Read the model definition and answer for the solid it produces. Units are mm, in the model's axes. Face numbers are marked on the shaded views. A direction names the side the tool comes from. Coordinates: 2 decimals unless noted, no trailing zeros. Order: outer loops, then holes, each group sorted by start corner. A loop starts at its lowest first (then second) coordinate and runs counter-clockwise, first axis right, second up. Notation, with made-up numbers: (-37, -7) -> (13, -7) arc R27 cw to (13, 28) -> close; hole circle Ø4 at (72, 86.5). An arc over 180 degrees is marked (long way). Answer as a JSON object with one key per item and string values. Group by question number.
1) Consider L1, parallel to X at y = -4.5, z = 1.95; L2, parallel to Y at x = 0, z = 1.3; L3, parallel to Y at x = 0, z = 4.2. Determine where each line is inside the solid, lowest interval first.
2) A tool of negligible diameter and unlimited length cuts with its end or side. For the marked faces 1 and 2, from which of +Z, -Z, +X, -X, +Y, -Y can it reach the whole face along a straight path? Write none if from no direction.
3) Section C-C on z = 2 is taken. Determine the outline of the cut face in (x, y), and give its area (3 significant figures).
4) Section D-D on y = -4.75 is taken. Determine the outline of the cut face in (x, z).
5) Determine the mould class of the marked faces 3, 4 and 5 for opening direction Z: released by +Z, released by -Z, zero draft, split by the parting line, or undercut.
6) Section B-B on y = 0 is taken. Determine the outline of the cut face in (x, z), and give its area (3 significant figures).
7) Section A-A on x = 0 is taken. Determine the outline of the cut face in (y, z), and give its area (3 significant figures).
8) Given pin 1 (2.5 mm diameter, centred on x = 2, y = 2, fed in from -Z), flat-ended and moving along its own axis, determine where the tip first touches the part or whether it passes through.
from build123d import *

# Parameters (mm, degrees)
ESBO_O6_R                  = 5.25
ESBO_O6_R_2                = 4.1
RESSALTO_EXTRUS_O3_DEPTH   = 4
ESBO_O7_R                  = 5.25
RESSALTO_EXTRUS_O4_DEPTH   = 0.5
ESBO_O9_R                  = 0.65
RESSALTO_EXTRUS_O5_DEPTH   = 1.2
ESBO_O12_R                 = 3
CORTE_EXTRUS_O5_DEPTH      = 10
RESSALTO_EXTRUS_O6_START   = 4
ESBO_O13_R                 = 4.1
ESBO_O13_R_2               = 3.85
RESSALTO_EXTRUS_O6_DEPTH   = 4
ESBO_O16_W                 = 2.665336127
ESBO_O16_H                 = 7.90902753
ESBO_O16_W_2               = 2.097265449
ESBO_O16_H_2               = 7.395164159
CORTE_EXTRUS_O7_DEPTH      = 10
ESBO_O15_W                 = 9
ESBO_O15_H                 = 11
ESBO_O15_R                 = 3.85
RESSALTO_EXTRUS_O7_DEPTH   = 4.5
CORTE_EXTRUS_O6_REACH      = 18.756
CORTE_EXTRUS_O6_END_RADIUS = 3.85
ESBO_O14_R                 = 0.5


with BuildPart() as part:
    # Esboço6 → Ressalto-extrusão3 (new body)
    with BuildSketch(Plane.XY):
        Circle(ESBO_O6_R)
        Circle(ESBO_O6_R_2, mode=Mode.SUBTRACT)
    extrude(amount=RESSALTO_EXTRUS_O3_DEPTH)

    # Esboço7 → Ressalto-extrusão4 (add)
    with BuildSketch(Plane.XY.offset(4)):
        Circle(ESBO_O7_R)
    extrude(amount=RESSALTO_EXTRUS_O4_DEPTH)

    # Esboço9 → Ressalto-extrusão5 (add)
    with BuildSketch(Plane(origin=(0, 0, 0), x_dir=(-1, 0, 0), z_dir=(0, 0, -1))):
        with Locations(Location((0, 4.75, 0), (0, 0, 132.158106499))):
            Circle(ESBO_O9_R)
        with Locations(Location((0, -4.75, 0), (0, 0, 227.841893501))):
            Circle(ESBO_O9_R)
    extrude(amount=RESSALTO_EXTRUS_O5_DEPTH)

    # Esboço12 → Corte-extrusão5 (cut)
    with BuildSketch(Plane(origin=(0, 0, 4), x_dir=(-1, 0, 0), z_dir=(0, 0, -1))):
        Circle(ESBO_O12_R)
    extrude(amount=-CORTE_EXTRUS_O5_DEPTH, mode=Mode.SUBTRACT)

    # Esboço13 → Ressalto-extrusão6 (add)
    with BuildSketch(Plane(origin=(0, 0, 4), x_dir=(-1, 0, 0), z_dir=(0, 0, -1)).offset(RESSALTO_EXTRUS_O6_START)):
        Circle(ESBO_O13_R)
        with Locations(Location((0, 0, 0), (0, 0, 180))):
            Circle(ESBO_O13_R_2, mode=Mode.SUBTRACT)
    extrude(amount=-RESSALTO_EXTRUS_O6_DEPTH)

    # Esboço16 → Corte-extrusão7 (cut)
    with BuildSketch(Plane(origin=(0, 0, 0), x_dir=(-1, 0, 0), z_dir=(0, 0, -1))):
        with Locations((5.832668063, -0.340062901)):
            Rectangle(ESBO_O16_W, ESBO_O16_H)
        with Locations((-5.548632725, -0.440601387)):
            Rectangle(ESBO_O16_W_2, ESBO_O16_H_2)
    extrude(amount=-CORTE_EXTRUS_O7_DEPTH, mode=Mode.SUBTRACT)

    # Esboço15 → Ressalto-extrusão7 (add)
    with BuildSketch(Plane(origin=(0, 0, 0), x_dir=(-1, 0, 0), z_dir=(0, 0, -1))):
        Rectangle(ESBO_O15_W, ESBO_O15_H)
        with Locations(Location((0, 0, 0), (0, 0, 180))):
            Circle(ESBO_O15_R, mode=Mode.SUBTRACT)
    extrude(amount=-RESSALTO_EXTRUS_O7_DEPTH)

    # Corte-extrusão6: up to this cylinder (the profile starts outside it)
    corte_extrus_o6_end = Plane(origin=(0, 0, 2), z_dir=(0, 0, 1)) * Cylinder(CORTE_EXTRUS_O6_END_RADIUS, 46.212, mode=Mode.PRIVATE)
    # Esboço14 → Corte-extrusão6 (cut, up to the surface)
    with BuildSketch(Plane(origin=(0, -10, 0), x_dir=(1, 0, 0), z_dir=(0, 1, 0)), mode=Mode.PRIVATE) as corte_extrus_o6_sk1:
        with Locations(Location((0, -2, 0), (0, 0, 90))):
            Circle(ESBO_O14_R)
    corte_extrus_o6_tool1 = extrude(corte_extrus_o6_sk1.sketch, amount=CORTE_EXTRUS_O6_REACH, mode=Mode.PRIVATE) - corte_extrus_o6_end
    add(corte_extrus_o6_tool1.solids().sort_by_distance((0, -10, 2))[0], mode=Mode.SUBTRACT)


solid = part.part
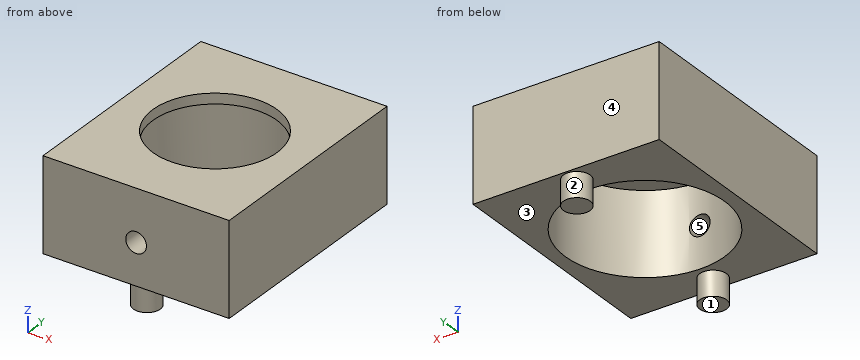
Worked answers:
{
 "1": {"L1": "x = -4.5 to -0.5, 0.5 to 4.5", "L2": "y = -5.5 to -3.85, 3.85 to 5.5", "L3": "y = -5.5 to -3, 3 to 5.5"},
 "2": {"face 1": "-Z, +X, -X, +Y, -Y", "face 2": "-Z"},
 "3": {"outline": "(-4.5, -5.5) -> (-0.5, -5.5) -> (-0.5, -3.82) arc R3.85 cw (long way) to (0.5, -3.82) -> (0.5, -5.5) -> (4.5, -5.5) -> (4.5, 5.5) -> (-4.5, 5.5) -> close", "area": "50.8 mm²"},
 "4": {"outline": "(-4.5, 0) -> (-0.65, 0) -> (-0.65, -1.2) -> (0.65, -1.2) -> (0.65, 0) -> (4.5, 0) -> (4.5, 4.5) -> (-4.5, 4.5) -> close; hole circle Ø1 at (0, 2)"},
 "5": {"face 3": "released by -Z", "face 4": "zero draft", "face 5": "undercut"},
 "6": {"outline": "(-4.5, 0) -> (-3.85, 0) -> (-3.85, 4) -> (-3, 4) -> (-3, 4.5) -> (-4.5, 4.5) -> close; (3, 4) -> (3.85, 4) -> (3.85, 0) -> (4.5, 0) -> (4.5, 4.5) -> (3, 4.5) -> close", "area": "6.70 mm²"},
 "7": {"outline": "(-5.5, 0) -> (-5.4, 0) -> (-5.4, -1.2) -> (-4.1, -1.2) -> (-4.1, 0) -> (-3.85, 0) -> (-3.85, 1.5) -> (-5.5, 1.5) -> close; (-5.5, 2.5) -> (-3.85, 2.5) -> (-3.85, 4) -> (-3, 4) -> (-3, 4.5) -> (-5.5, 4.5) -> close; (3, 4) -> (3.85, 4) -> (3.85, 0) -> (4.1, 0) -> (4.1, -1.2) -> (5.4, -1.2) -> (5.4, 0) -> (5.5, 0) -> (5.5, 4.5) -> (3, 4.5) -> close", "area": "17.2 mm²"},
 "8": {"pin 1": "stops at z = 0"}
}
